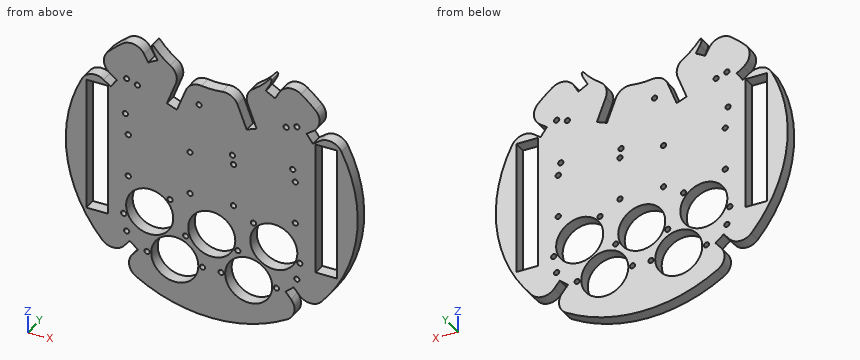
```python
from build123d import *

# Parameters (mm, degrees)
BOSS_EXTRUDE3_OUTLINE_R   = 1.35
BOSS_EXTRUDE3_OUTLINE_W   = 11
BOSS_EXTRUDE3_OUTLINE_H   = 69
BOSS_EXTRUDE3_OUTLINE_R_2 = 12.095
BOSS_EXTRUDE3_DEPTH       = 6.35
FILLET5_R                 = 0.5


# Read off the part's stored shape, not the designer's step: Boss-Extrude3
with BuildPart() as part:
    # Boss-Extrude3 outline → Boss-Extrude3 (new body)
    with BuildSketch(Plane(origin=(0, 0, 0), x_dir=(1, 0, 0), z_dir=(0, 1, 0))):
        with BuildLine():
            ThreePointArc((30.845959646, -64.038266509), (30.722917613, -61.793165345), (29.939937248, -59.685427143))
            Line((29.939937248, -59.685427143), (27.754427747, -55.742664454))
            ThreePointArc((27.754427747, -55.742664454), (30.189085526, -54.462574444), (32.564835967, -53.076212737))
            Line((32.564835967, -53.076212737), (34.750345491, -57.018976288))
            ThreePointArc((34.750345491, -57.018976288), (39.797694407, -60.728851606), (45.899993549, -59.314337155))
            ThreePointArc((45.899993549, -59.314337155), (49.682691748, -56.183895741), (53.252452412, -52.812652955))
            ThreePointArc((53.252452412, -52.812652955), (55.400241506, -46.895968251), (52.284336639, -41.426846498))
            Line((52.284336639, -41.426846498), (48.694399386, -38.812476969))
            ThreePointArc((48.694399386, -38.812476969), (50.363701809, -36.620355543), (51.934395763, -34.35653412))
            Line((51.934395763, -34.35653412), (55.532494673, -36.970706015))
            ThreePointArc((55.532494673, -36.970706015), (61.694807292, -38.244055423), (66.658022594, -34.375979751))
            ThreePointArc((66.658022594, -34.375979751), (74.442134424, 9.130641951), (56.374397975, 49.466425512))
            ThreePointArc((56.374397975, 49.466425512), (50.654117331, 52.01932544), (44.991624855, 49.340690033))
            Line((44.991624855, 49.340690033), (42.093955335, 45.887381973))
            ThreePointArc((42.093955335, 45.887381973), (40.026384455, 47.701587473), (37.880710897, 49.422713826))
            Line((37.880710897, 49.422713826), (40.778380417, 52.876021886))
            ThreePointArc((40.778380417, 52.876021886), (42.433039833, 58.917628535), (38.925607882, 64.107698843))
            ThreePointArc((38.925607882, 64.107698843), (0, 75), (-38.925607882, 64.107698843))
            ThreePointArc((-38.925607882, 64.107698843), (-42.433039833, 58.917628535), (-40.778380417, 52.876021886))
            Line((-40.778380417, 52.876021886), (-37.880710897, 49.422713826))
            ThreePointArc((-37.880710897, 49.422713826), (-40.026384455, 47.701587473), (-42.093955335, 45.887381973))
            Line((-42.093955335, 45.887381973), (-44.991624855, 49.340690033))
            ThreePointArc((-44.991624855, 49.340690033), (-50.654117331, 52.01932544), (-56.374397975, 49.466425512))
            ThreePointArc((-56.374397975, 49.466425512), (-74.442134424, 9.130641951), (-66.658022831, -34.375979873))
            ThreePointArc((-66.658022831, -34.375979873), (-61.694807292, -38.244055423), (-55.532494673, -36.970706015))
            Line((-55.532494673, -36.970706015), (-51.934395763, -34.35653412))
            ThreePointArc((-51.934395763, -34.35653412), (-50.363701809, -36.620355543), (-48.694399386, -38.812476969))
            Line((-48.694399386, -38.812476969), (-52.284336639, -41.426846498))
            ThreePointArc((-52.284336639, -41.426846498), (-55.400241506, -46.895968251), (-53.252452412, -52.812652955))
            ThreePointArc((-53.252452412, -52.812652955), (-49.682691748, -56.183895741), (-45.899993549, -59.314337155))
            ThreePointArc((-45.899993549, -59.314337155), (-39.797694407, -60.728851606), (-34.750345491, -57.018976288))
            Line((-34.750345491, -57.018976288), (-32.564835967, -53.076212737))
            ThreePointArc((-32.564835967, -53.076212737), (-30.189085526, -54.462574444), (-27.754427747, -55.742664454))
            Line((-27.754427747, -55.742664454), (-29.939937248, -59.685427143))
            ThreePointArc((-29.939937248, -59.685427143), (-30.722917613, -61.793165345), (-30.845959646, -64.038266509))
            ThreePointArc((-30.845959646, -64.038266509), (-26.466137741, -58.99482374), (-21.272807595, -54.79381471))
            ThreePointArc((-21.272807595, -54.79381471), (-18.309924074, -50.834725832), (-18.455489673, -45.891864903))
            Line((-18.455489673, -45.891864903), (-23.054134296, -33.922453045))
            Line((-23.054134296, -33.922453045), (-17.920018766, -31.949927322))
            Line((-17.920018766, -31.949927322), (-13.321374143, -43.91933918))
            ThreePointArc((-13.321374143, -43.91933918), (-10.119925368, -47.688130663), (-5.268365652, -48.644912678))
            ThreePointArc((-5.268365652, -48.644912678), (0, -48.279128696), (5.268365652, -48.644912678))
            ThreePointArc((5.268365652, -48.644912678), (10.119925368, -47.688130663), (13.321374143, -43.91933918))
            Line((13.321374143, -43.91933918), (17.920018766, -31.949927322))
            Line((17.920018766, -31.949927322), (23.054134296, -33.922453045))
            Line((23.054134296, -33.922453045), (18.455489673, -45.891864903))
            ThreePointArc((18.455489673, -45.891864903), (18.309924074, -50.834725832), (21.272807595, -54.79381471))
            ThreePointArc((21.272807595, -54.79381471), (26.466137741, -58.99482374), (30.845959646, -64.038266509))
        make_face()
        with Locations((-43.735655662, -41.075447944)):
            Circle(BOSS_EXTRUDE3_OUTLINE_R, mode=Mode.SUBTRACT)
        with Locations((-38.234289702, -39.23697625)):
            Circle(BOSS_EXTRUDE3_OUTLINE_R, mode=Mode.SUBTRACT)
        with Locations((-6.55476095, -38.026099982)):
            Circle(BOSS_EXTRUDE3_OUTLINE_R, mode=Mode.SUBTRACT)
        with Locations((-44.385223141, -22.074211772)):
            Circle(BOSS_EXTRUDE3_OUTLINE_R, mode=Mode.SUBTRACT)
        with Locations((-58.910067426, 0.102907352)):
            Rectangle(BOSS_EXTRUDE3_OUTLINE_W, BOSS_EXTRUDE3_OUTLINE_H, mode=Mode.SUBTRACT)
        with Locations((-42.910067426, -11.1)):
            Circle(BOSS_EXTRUDE3_OUTLINE_R, mode=Mode.SUBTRACT)
        with Locations((-11.160067426, -11.1)):
            Circle(BOSS_EXTRUDE3_OUTLINE_R, mode=Mode.SUBTRACT)
        with Locations((38.234289702, -39.23697625)):
            Circle(BOSS_EXTRUDE3_OUTLINE_R, mode=Mode.SUBTRACT)
        with Locations((43.735655662, -41.075447944)):
            Circle(BOSS_EXTRUDE3_OUTLINE_R, mode=Mode.SUBTRACT)
        with Locations((10.597026674, -15.930038136)):
            Circle(BOSS_EXTRUDE3_OUTLINE_R, mode=Mode.SUBTRACT)
        with Locations((11.160067426, -11.1)):
            Circle(BOSS_EXTRUDE3_OUTLINE_R, mode=Mode.SUBTRACT)
        with Locations((41.601681906, -17.457756634)):
            Circle(BOSS_EXTRUDE3_OUTLINE_R, mode=Mode.SUBTRACT)
        with Locations((42.910067426, -11.1)):
            Circle(BOSS_EXTRUDE3_OUTLINE_R, mode=Mode.SUBTRACT)
        with Locations((58.910067426, 0.102907352)):
            Rectangle(BOSS_EXTRUDE3_OUTLINE_W, BOSS_EXTRUDE3_OUTLINE_H, mode=Mode.SUBTRACT)
        with Locations((-42.910067426, 11.1)):
            Circle(BOSS_EXTRUDE3_OUTLINE_R, mode=Mode.SUBTRACT)
        with Locations((-45.242610731, 31.997163897)):
            Circle(BOSS_EXTRUDE3_OUTLINE_R, mode=Mode.SUBTRACT)
        with Locations((-21.451773633, 17.449398418)):
            Circle(BOSS_EXTRUDE3_OUTLINE_R, mode=Mode.SUBTRACT)
        with Locations((-11.160067426, 11.1)):
            Circle(BOSS_EXTRUDE3_OUTLINE_R, mode=Mode.SUBTRACT)
        with Locations((-31.895736851, 27.096933482)):
            Circle(BOSS_EXTRUDE3_OUTLINE_R_2, mode=Mode.SUBTRACT)
        with Locations((-13.346873881, 34.693819966)):
            Circle(BOSS_EXTRUDE3_OUTLINE_R, mode=Mode.SUBTRACT)
        with Locations((-43.735655662, 41.075447944)):
            Circle(BOSS_EXTRUDE3_OUTLINE_R, mode=Mode.SUBTRACT)
        with Locations((-33.21799214, 49)):
            Circle(BOSS_EXTRUDE3_OUTLINE_R, mode=Mode.SUBTRACT)
        with Locations((-19, 49)):
            Circle(BOSS_EXTRUDE3_OUTLINE_R_2, mode=Mode.SUBTRACT)
        with Locations((-4.78200786, 49)):
            Circle(BOSS_EXTRUDE3_OUTLINE_R, mode=Mode.SUBTRACT)
        with Locations((11.160067426, 11.1)):
            Circle(BOSS_EXTRUDE3_OUTLINE_R, mode=Mode.SUBTRACT)
        with Locations((21.451773633, 17.449398418)):
            Circle(BOSS_EXTRUDE3_OUTLINE_R, mode=Mode.SUBTRACT)
        with Locations((0, 29.793589551)):
            Circle(BOSS_EXTRUDE3_OUTLINE_R_2, mode=Mode.SUBTRACT)
        with Locations((13.346873881, 34.693819966)):
            Circle(BOSS_EXTRUDE3_OUTLINE_R, mode=Mode.SUBTRACT)
        with Locations((31.895736851, 27.096933482)):
            Circle(BOSS_EXTRUDE3_OUTLINE_R_2, mode=Mode.SUBTRACT)
        with Locations((42.910067426, 11.1)):
            Circle(BOSS_EXTRUDE3_OUTLINE_R, mode=Mode.SUBTRACT)
        with Locations((45.242610731, 31.997163897)):
            Circle(BOSS_EXTRUDE3_OUTLINE_R, mode=Mode.SUBTRACT)
        with Locations((4.78200786, 49)):
            Circle(BOSS_EXTRUDE3_OUTLINE_R, mode=Mode.SUBTRACT)
        with Locations((19, 49)):
            Circle(BOSS_EXTRUDE3_OUTLINE_R_2, mode=Mode.SUBTRACT)
        with Locations((33.21799214, 49)):
            Circle(BOSS_EXTRUDE3_OUTLINE_R, mode=Mode.SUBTRACT)
        with Locations((43.735655662, 41.075447944)):
            Circle(BOSS_EXTRUDE3_OUTLINE_R, mode=Mode.SUBTRACT)
    extrude(amount=BOSS_EXTRUDE3_DEPTH)

    # Fillet5
    fillet5_edges = [part.edges().sort_by_distance(p)[0] for p in [
        (30.845959646, 3.175, 64.038266509),
        (-30.845959646, 3.175, 64.038266509),
    ]]
    fillet(fillet5_edges, radius=FILLET5_R)


solid = part.part
```
Geometry: final body of the model. Coordinates: model frame, mm. Round coordinates to 2 decimals unless told otherwise and drop trailing zeros. Order: outer loops, then holes, each group sorted by start corner. A loop starts at its lowest first (then second) coordinate and runs counter-clockwise, first axis right, second up. Notation, with made-up numbers: (4.5, -14) - (39.5, -14) arc R10 cw to (39.5, -6) - close; hole circle Ø6 at (-13.5, 53.5). An arc over 180 degrees is marked (long way). Write item = value, one per line. Start each with the question number.
Q1. Cut plane A-A on z = 26. Return the cut outline in (x, y), and give its area (3 significant figures).
Q2. Cut plane B-B on y = 3. Give the number of separate pieces and of enclosed holes in the cut face, and give its area (3 significant figures).
Q3. Ray query, line 1 (X direction, y = 0.5, z = -22); line 2 (Z direction, x = -6.5, y = 0.5); line 3 (X direction, y = 6, z = 4). Return the intervals inside material, ascending. Write a range as from..to.
Q4. Pin query (flat end, axial travel): pin 1 (1.9 mm diameter, centred on y = 3, z = -14.5, fed in from +X); pin 2 (3 mm diameter, centred on y = 1, z = -52, fed in from +X); pin 3 (3 mm diameter, centred on x = 37.5, y = 5.5, fed in from -Z). Return the tip coordinate at first contact, or that it passes through.
Outcome:
q1.outline = (-70.35, 0) - (-64.41, 0) - (-64.41, 6.35) - (-70.35, 6.35) - close; (-53.41, 0) - (53.41, 0) - (53.41, 6.35) - (-53.41, 6.35) - close; (64.41, 0) - (70.35, 0) - (70.35, 6.35) - (64.41, 6.35) - close
q1.area = 754 mm^2
q2.separate_pieces = 1
q2.enclosed_holes = 35
q2.area = 11,600 mm^2
q3.line_1 = -71.7..-64.41, -53.41..-42.86, -20.93..-9.25, 9.25..20.93, 42.86..53.41, 64.41..71.7
q3.line_2 = -74.72..-39.99, -19.59..36.68, 39.37..48.72
q3.line_3 = -74.89..-64.41, -53.41..53.41, 64.41..74.89
q4.pin_1 = 73.77
q4.pin_2 = 55.26
q4.pin_3 = -65.8
